Model file for the job. Use its own axes, mm. A direction names the side the tool comes from. Give positions to 0.01 mm unless a question says otherwise; leave off trailing zeros. Write each loop counter-clockwise with the first axis right and the second up, starting at its lowest first coordinate (ties: lowest second). Pieces come first, ordered by that corner, then holes. Notation, with made-up numbers: (19, 2.5) - (60, 2.5) arc R24 cw to (60, 38.5) - close; hole circle Ø4 at (-23.5, 89). An arc over 180 degrees is marked (long way). One line per item, written item: value. Start each with the question number.
(1) 3-axis set-ups, long thin cutter, end or side, ignore diameter. For faces 1 (the face through (-26.677, 21.036, -22.536)), 2 (the face through (-31.75, 85, -2)), 3 (the face through (-15.653, 36.007, -35.744)): which of +Z, -Z, +X, -X, +Y, -Y reach the whole face in a straight line?
(2) Probe L1, parallel to Y at x = -28, z = -28 (3 decimals); L2, parallel to Y at x = -9.5, z = -3; L3, parallel to Y at x = -15, z = -32 (3 decimals). List the from-to ranges inside material, lowest first.
(3) Mould opens along Z. For faces 4 (the face through (-16, 64, -44.45)), 5 (the face through (-15.65, 102.75, -36.35)), 6 (the face through (-16.1, 39.08, -3.91)), 7 (the face through (-31.75, 5, -22)) say: pulls with the +Z half, pulls with the -Z half, needs draft (parallel to the pull), parting line crosses it, or undercut.
(4) Drop a flat-ended pin along its axis: P1, Ø2, axis at x = -5.5, z = -5.5, coming from the -Y side. Give the stop position or say it passes through.
(5) Cut at C-C, the plane y = 93.5. List the corners of the cut face in (x, z) (3 decimals), and give its area (3 significant figures).
(6) Cut at B-B, the plane x = -19.5. State how many separate pieces and enclosed holes the cut face has, and give its area (3 significant figures).
Autodesk Inventor part; units mm, degrees
ref_plane "YZ Plane" through (0, 0, 0) normal (1, 0, 0) x (0, 1, 0)
ref_plane "XZ Plane" through (0, 0, 0) normal (0, 1, 0) x (-1, 0, 0)
ref_plane "XY Plane" through (0, 0, 0) normal (0, 0, 1) x (1, 0, 0)
sketch "Sketch1" plane through (0, 0, 0) normal (1, 0, 0) x (0, 1, 0)
  line L0 (0, 0) -> (127, 0)
  line L1 (127, 0) -> (127, -44.45)
  line L2 (127, -44.45) -> (0, -44.45)
  line L3 (0, -44.45) -> (0, 0)
  line L4 (15.875, -44.45) -> (15.875, 0) construction
  line L5 (28.575, -44.45) -> (28.575, 0)
  line L6 (28.575, -44.45) -> (127, 0) construction
  line L7 (127, -44.45) -> (28.575, 0) construction
  arc A0 (28.575, -4.7625) -> (33.3375, 0) centre (33.3375, -4.7625) ccw
  circle A1 centre (33.3375, -4.7625) radius 3.3655
  line L8 (28.575, -22.225) -> (127, -22.225) construction
  line L9 (37.8276, -41.275) -> (98.425, -41.275)
  line L10 (98.425, -41.275) -> (98.425, -3.175)
  line L11 (98.425, -3.175) -> (37.8276, -3.175)
  arc A2 (33.3375, -44.45) -> (28.575, -39.6875) centre (33.3375, -39.6875) ccw
  circle A3 centre (33.3375, -39.6875) radius 3.3655
  circle A4 centre (103.1875, -39.6875) radius 4.7625 construction
  circle A5 centre (103.1875, -39.6875) radius 3.3655
  circle A6 centre (103.1875, -4.7625) radius 4.7625 construction
  circle A7 centre (103.1875, -4.7625) radius 3.3655
  point P0 (77.7875, -22.225)
  dimension "d0" = 127
  dimension "d1" = 44.45
  dimension "d2" = 15.875
  dimension "d4" = 12.7
  dimension "d5" = 9.525
  dimension "d6" = 6.731
  dimension "d7" = 3.175
  dimension "d8" = 3.175
  dimension "d9" = 69.85
  dimension "d10" = 9.525
  dimension "d11" = 6.731
extrude "Extrusion1" add sketch "Sketch1" against normal blind 31.75 contours L0 L5 L2 L3 | L0 A0 L5 | L0 L1 L2 A2 L9 L10 L11 A0 | L5 A2 L2
fillet "Fillet1" radius 3.175 6 edges at (-15.875, 28.575, -39.6875) (-15.875, 37.8276, -41.275) (-15.875, 98.425, -41.275) (-15.875, 98.425, -3.175) (-15.875, 37.8276, -3.175) (-15.875, 28.575, -4.7625)
sketch "Sketch2" plane through (0, 0, 0) normal (0, 0, 1) x (1, 0, 0)
  line L0 (0, 0) -> (-31.75, 0) construction
  line L1 (-15.875, 0) -> (-15.875, 127) construction
  line L2 (0, 127) -> (-31.75, 127) construction
  circle A0 centre (-15.875, 15.875) radius 11.5
  line L3 (-38.875, 11.1125) -> (-15.875, 11.1125)
  line L4 (-15.875, 11.1125) -> (-15.875, 20.6375)
  line L5 (-15.875, 20.6375) -> (-38.875, 20.6375)
  line L6 (-38.875, 20.6375) -> (-38.875, 11.1125)
  line L7 (-38.875, 11.1125) -> (-15.875, 20.6375) construction
  line L8 (-15.875, 11.1125) -> (-38.875, 20.6375) construction
  line L9 (-15.875, 15.875) -> (-27.375, 15.875) construction
  point P0 (-26.3425, 11.1125)
  point P1 (-26.3425, 20.6375)
  dimension "d15" = 23
  dimension "d16" = 15.875
  dimension "d17" = 9.525
extrude "Extrusion2" cut sketch "Sketch2" against normal through all
fillet "Fillet2" radius 3.175 2 edges at (-26.3425, 11.1125, -22.225) (-26.3425, 20.6375, -22.225)
equation "\"d8\" = d7"
properties part number "Pod" material "Rubber, Silicone"
Answers follow:
1. face 1: +Z, -Z
1. face 2: +Z, -Z, -X, +Y, -Y
1. face 3: +X, -X
2. L1: y = 0 to 11.105, 20.645 to 28.575, 98.425 to 127
2. L2: y = 0 to 6.3, 25.45 to 30.47, 36.2 to 100.32, 106.05 to 127
2. L3: y = 0 to 4.408, 27.342 to 28.576, 98.425 to 127
3. face 4: pulls with the -Z half
3. face 5: undercut
3. face 6: undercut
3. face 7: needs draft
4. P1: stops at y = 0
5. outline: (-31.75, -44.45) - (0, -44.45) - (0, -41.275) - (-31.75, -41.275) - close; (-31.75, -3.175) - (0, -3.175) - (0, 0) - (-31.75, 0) - close
5. area: 202 mm²
6. separate pieces: 2
6. enclosed holes: 5
6. area: 1,990 mm²
